Study the drawing (mm; zero at the part's minimum x, y, z) and answer. Give positions to 0.01 mm unless a question says otherwise; leave off trailing zeros. Loops run counter-clockwise (first coordinate to the right, second up) from the corner with the lowest first, then second, coordinate; pieces in that order, holes last. Notation, with made-up numbers: (12, -30.5) - (63, -30.5) arc R20 ccw to (63, -9.5) - close; hole circle Ø9 at (66, -29.5). An arc over 180 degrees is marked (long way). Write item = value, one per line. Start each with the question number.
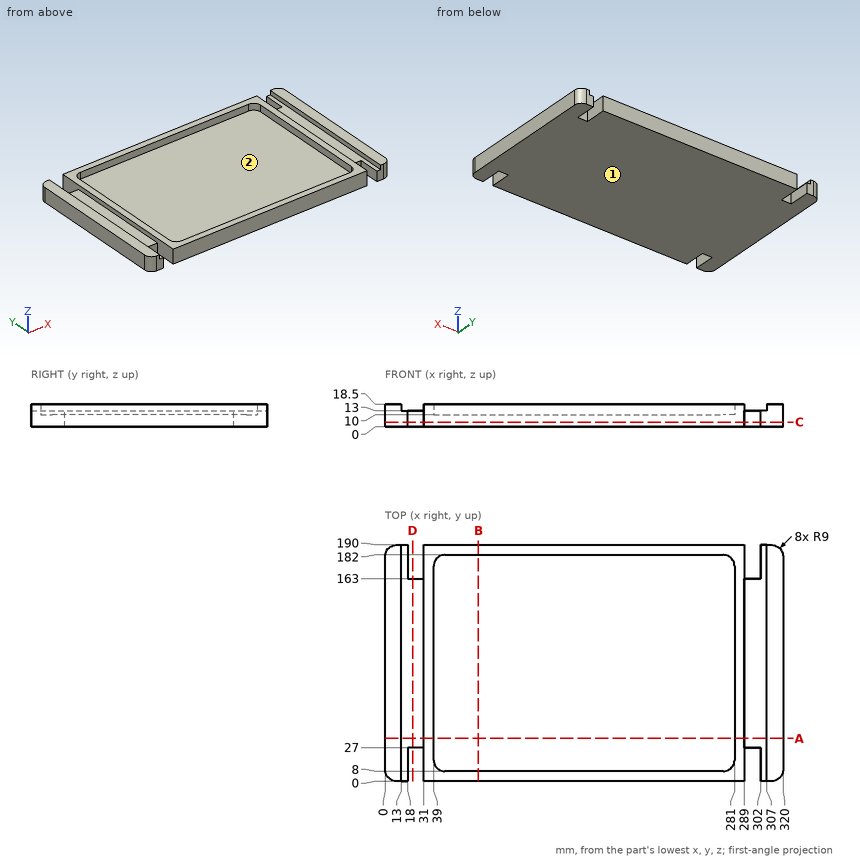
1. For a pull along Y with two mould halves and no side action, classify the marked faces 1 and 2 as released by +Y, released by -Y, zero draft, split by the parting line, or undercut.
2. Consider line 1 along X through (y, z) = (84, 15.5); line 2 along X through (y, z) = (175, 9.75); line 3 along X through (y, z) = (26, 12.75). Determine where each line is inside the solid, lowest interval first. Write a range as [from, to].
3. A cutting plane is placed at D-D on x = 22. Give the vertices of the cut face in (y, z).
4. Given P1, Ø4, axis at x = 293, z = 6, coming from the -Y side, flat-ended and moving along its own axis, determine where the tip first touches the part or whether it passes through.
5. A cutting plane is placed at A-A on y = 34.5. Give the vertices of the cut face in (x, z), and give its area (4 significant figures).
6. A cutting plane is placed at B-B on x = 75. Give the vertices of the cut face in (y, z).
7. A cutting plane is placed at C-C on z = 4. Give the vertices of the cut face in (x, y).
Reply:
q1.face_1 = zero draft
q1.face_2 = undercut
q2.line_1 = [0, 13], [31, 39], [281, 289], [307, 320]
q2.line_2 = [0, 18], [31, 289], [302, 320]
q2.line_3 = [0, 18], [31, 39], [281, 289], [302, 320]
q3.outline = (27, 0) - (163, 0) - (163, 13) - (27, 13) - close
q4.P1 = 27
q5.outline = (0, 0) - (320, 0) - (320, 18.5) - (307, 18.5) - (307, 13) - (289, 13) - (289, 18.5) - (281, 18.5) - (281, 10) - (39, 10) - (39, 18.5) - (31, 18.5) - (31, 13) - (13, 13) - (13, 18.5) - (0, 18.5) - close
q5.area = 3,665 mm^2
q6.outline = (0, 0) - (190, 0) - (190, 18.5) - (182, 18.5) - (182, 10) - (8, 10) - (8, 18.5) - (0, 18.5) - close
q7.outline = (0, 9) arc R9 ccw to (9, 0) - (18, 0) - (18, 27) - (31, 27) - (31, 0) - (289, 0) - (289, 27) - (302, 27) - (302, 0) - (311, 0) arc R9 ccw to (320, 9) - (320, 181) arc R9 ccw to (311, 190) - (302, 190) - (302, 163) - (289, 163) - (289, 190) - (31, 190) - (31, 163) - (18, 163) - (18, 190) - (9, 190) arc R9 ccw to (0, 181) - close
